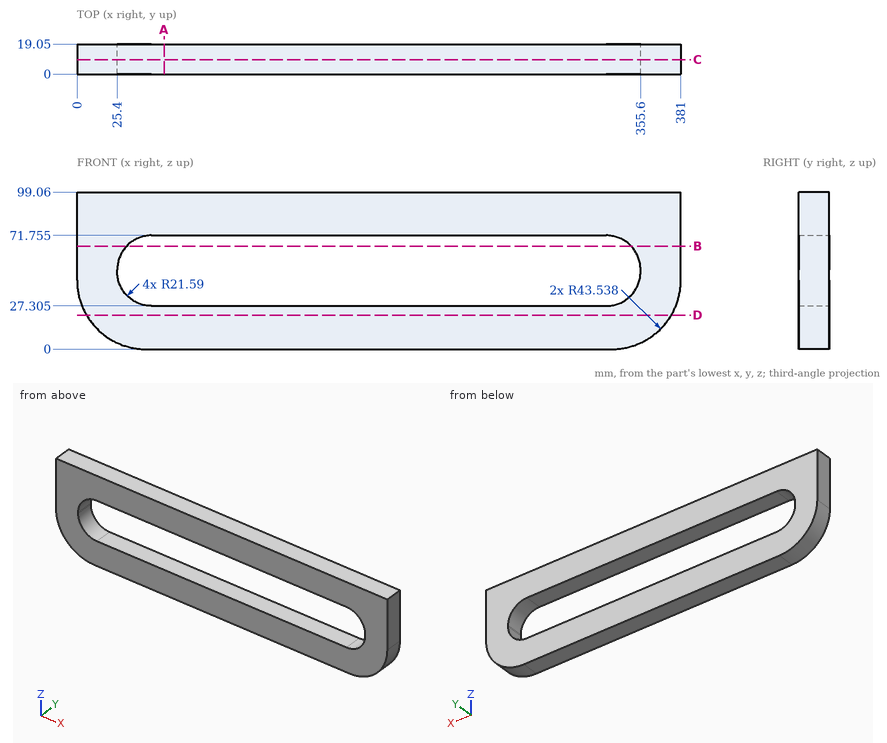
Geometry: see drawing. Coordinates: mm, zero at the bounding-box minimum. Give positions to 0.01 mm unless a question says otherwise; leave off trailing zeros. Loops run counter-clockwise (first coordinate to the right, second up) from the corner with the lowest first, then second, coordinate; pieces in that order, holes last. Notation, with made-up numbers: (-28.5, 71) -> (-20.5, 71) arc R8 cw to (-20.5, 77) -> close; hole circle Ø11 at (60.25, -30). An arc over 180 degrees is marked (long way). Use one line per item in the form item = value.
Item 1: Section query B-B on z = 65. Output: boundary loops of the cut face in (x, y), and give its area (3 significant figures).
A:
outline = (0, 0) -> (31.3, 0) -> (31.3, 19.05) -> (0, 19.05) -> close; (349.7, 0) -> (381, 0) -> (381, 19.05) -> (349.7, 19.05) -> close
area = 1,190 mm^2
Item 2: Section query D-D on z = 21.5. Output: boundary loops of the cut face in (x, y).
A:
outline = (5.99, 0) -> (375.01, 0) -> (375.01, 19.05) -> (5.99, 19.05) -> close
Item 3: Section query C-C on y = 9.25. Output: boundary loops of the cut face in (x, z) (3 decimals), and give its area (3 significant figures).
A:
outline = (0, 43.538) arc R43.538 ccw to (43.538, 0) -> (337.462, 0) arc R43.538 ccw to (381, 43.538) -> (381, 99.06) -> (0, 99.06) -> close; hole (25.4, 48.895) arc R21.59 ccw to (46.99, 27.305) -> (334.01, 27.305) arc R21.59 ccw to (355.6, 48.895) -> (355.6, 50.165) arc R21.59 ccw to (334.01, 71.755) -> (46.99, 71.755) arc R21.59 ccw to (25.4, 50.165) -> close
area = 22,700 mm^2
Item 4: Section query A-A on x = 55. Output: boundary loops of the cut face in (y, z) (3 decimals).
A:
outline = (0, 0) -> (19.05, 0) -> (19.05, 27.305) -> (0, 27.305) -> close; (0, 71.755) -> (19.05, 71.755) -> (19.05, 99.06) -> (0, 99.06) -> close
Item 5: Line query: probe 1 along Z at (x, y) = (323, 17) (3 decimals); probe 2 along Z at (x, y) = (347, 3.5); probe 3 along X at (y, z) = (3, 62). Output: solid intervals per line, ascending.
A:
probe_1 = 0 to 27.305, 71.755 to 99.06
probe_2 = 1.06 to 31.65, 67.41 to 99.06
probe_3 = 0 to 28.93, 352.07 to 381
